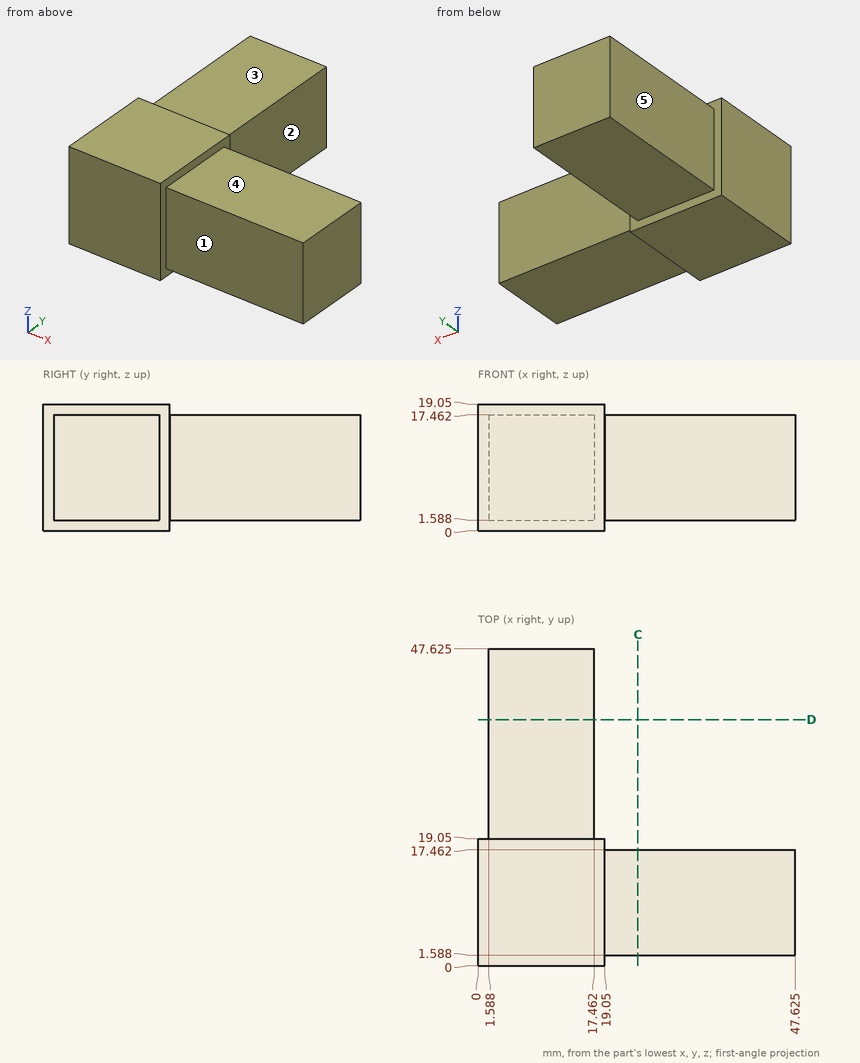
Can you work these out from the drawing? Everything is in mm from the part's minimum corner. A direction names the side the tool comes from. Give positions to 0.01 mm unless a question says otherwise; leave off trailing zeros. Loops run counter-clockwise (first coordinate to the right, second up) from the corner with the lowest first, then second, coordinate; pieces in that order, holes last. Notation, with made-up numbers: (-2.5, -40) -> (10.5, -40) arc R19 ccw to (10.5, -24) -> close; hole circle Ø7 at (-2, 19). An arc over 180 degrees is marked (long way). Return JSON: item names as keys, results as strings.
Q1. On a 3-axis mill with a long thin cutter (end or side, diameter ignored), from which of +Z, -Z, +X, -X, +Y, -Y can I reach the whole of each face in a straight line? I mean the marked faces 1, 2, 3, 4 and 5. Say none if no direction works.
Checks:
{"face 1": "+Z, -Z, +X, -Y", "face 2": "+Z, -Z, +X, +Y", "face 3": "+Z, +X, -X, +Y", "face 4": "+Z, +X, +Y, -Y", "face 5": "+Z, -Z, -X, +Y"}
Q2. I want a section at C-C, the plane x = 24. List the corners of the cut face in (y, z) for me.
Checks:
{"outline": "(1.59, 1.59) -> (17.46, 1.59) -> (17.46, 17.46) -> (1.59, 17.46) -> close"}
Q3. For pin 1 Ø1.5 at (x, z) = (13, 11) entering from -Y; pin 2 Ø8 at (x, y) = (37.5, 10) entering from +Z; pin 3 Ø2 at (y, z) = (40.5, 7) entering from +X; pin 4 Ø1.5 at (x, z) = (19, 8) entering from +Y, each with a flat end and sliding along its axis, tell me the tip position at first contact or that it passes through.
Checks:
{"pin 1": "stops at y = 0", "pin 2": "stops at z = 17.46", "pin 3": "stops at x = 17.46", "pin 4": "stops at y = 19.05"}
Q4. I need wall thicknesses on probe 1 along X at (y, z) = (29.5, 13.5). Which ranges of the line are inside material? Lowest first, please.
Checks:
{"probe 1": "x = 1.59 to 17.46"}
